from build123d import *
from build123d import SkipClean  # not in build123d's __all__

# Parameters (mm, degrees)
F0_R     = 6.1
F0_R_2   = 5
F1_DEPTH = 0.8
F2_R     = 6.1
F2_R_2   = 5.45
F3_DEPTH = 2.5
F4_R     = 5.45
F4_R_2   = 4.65
F5_DEPTH = 0.8
F7_DEPTH = 1.4
F9_DEPTH = 0.4


with BuildPart() as f1:
    # F0 (on Front) → F1 (new body)
    with BuildSketch(Plane.XZ):
        Circle(F0_R)
        Circle(F0_R_2, mode=Mode.SUBTRACT)
        Circle(F0_R_2)
    extrude(amount=F1_DEPTH)

    # F2 (on face) → F3 (join)
    with BuildSketch(Plane.XZ.offset(0.8)):
        Circle(F2_R)
        Circle(F2_R_2, mode=Mode.SUBTRACT)
    extrude(amount=F3_DEPTH)

    # F4 (on face) → F5 (join)
    with BuildSketch(Plane.XZ.offset(0.8)):
        Circle(F4_R)
        Circle(F4_R_2, mode=Mode.SUBTRACT)
    extrude(amount=F5_DEPTH)

    # F6 (on face) → F7 (cut)
    with BuildSketch(Plane.XZ.offset(3.3)):
        with BuildLine():
            Line((-1.2, -5.9808026217), (-1.6, -5.2098464469))
            ThreePointArc((-1.6, -5.2098464469), (-2.3813713563, -4.9022005735), (-3.1062049616, -4.4781682345))
            Line((-3.1062049616, -4.4781682345), (-2.555971444, -5.5386830544))
            ThreePointArc((-2.555971444, -5.5386830544), (-1.8909515594, -5.7995087895), (-1.2, -5.9808026217))
        make_face()
        with BuildLine():
            ThreePointArc((3.1062049616, -4.4781682345), (2.3813713563, -4.9022005735), (1.6, -5.2098464469))
            Line((1.6, -5.2098464469), (1.2, -5.9808026217))
            ThreePointArc((1.2, -5.9808026217), (1.8909515594, -5.7995087895), (2.555971444, -5.5386830544))
            Line((2.555971444, -5.5386830544), (3.1062049616, -4.4781682345))
        make_face()
    extrude(amount=-F7_DEPTH, mode=Mode.SUBTRACT)

    # F8 (on face) → F9 (join)
    with BuildSketch(Plane.XZ.offset(3.3)):
        with BuildLine():
            ThreePointArc((-1.6, -5.2098464469), (-2.3813713563, -4.9022005735), (-3.1062049616, -4.4781682345))
            Line((-3.1062049616, -4.4781682345), (-2.555971444, -5.5386830544))
            ThreePointArc((-2.555971444, -5.5386830544), (-1.8909515594, -5.7995087895), (-1.2, -5.9808026217))
            Line((-1.2, -5.9808026217), (-1.6, -5.2098464469))
        make_face()
        with BuildLine():
            Line((2.555971444, -5.5386830544), (3.1062049616, -4.4781682345))
            ThreePointArc((3.1062049616, -4.4781682345), (2.3813713563, -4.9022005735), (1.6, -5.2098464469))
            Line((1.6, -5.2098464469), (1.2, -5.9808026217))
            ThreePointArc((1.2, -5.9808026217), (1.8909515594, -5.7995087895), (2.555971444, -5.5386830544))
        make_face()
    with SkipClean():  # cleaning this boolean's faces spoils the solid; the shape is the same uncleaned
        extrude(amount=-F9_DEPTH)


solid = f1.part
CAD build for the part. Positions are in the model's coordinates, mm. A direction names the side the tool comes from. Give positions to 0.01 mm unless a question says otherwise; leave off trailing zeros. Write each loop counter-clockwise with the first axis right and the second up, starting at its lowest first coordinate (ties: lowest second). Pieces come first, ordered by that corner, then holes. Notation, with made-up numbers: (-25.5, 77.5) -> (17.5, 77.5) arc R38 ccw to (17.5, 115.5) -> close; hole circle Ø10 at (0, 62). An arc over 180 degrees is marked (long way). Return JSON: item names as keys, results as strings.
Item 1: Band-saw the part on D-D (x = 0). List the corners of the cut face in (y, z), then the cut area to 3 significant figures.
Answer below:
{"outline": "(-3.3, -6.1) -> (0, -6.1) -> (0, 6.1) -> (-3.3, 6.1) -> (-3.3, 5.45) -> (-1.6, 5.45) -> (-1.6, 4.65) -> (-0.8, 4.65) -> (-0.8, -4.65) -> (-1.6, -4.65) -> (-1.6, -5.45) -> (-3.3, -5.45) -> close", "area": "14.3 mm2"}
Item 2: Band-saw the part on B-B (z = 0). List the corners of the cut face in (x, y), then the cut area to 3 significant figures.
Answer below:
{"outline": "(-6.1, -3.3) -> (-5.45, -3.3) -> (-5.45, -1.6) -> (-4.65, -1.6) -> (-4.65, -0.8) -> (4.65, -0.8) -> (4.65, -1.6) -> (5.45, -1.6) -> (5.45, -3.3) -> (6.1, -3.3) -> (6.1, 0) -> (-6.1, 0) -> close", "area": "14.3 mm2"}
Item 3: Band-saw the part on C-C (x = -2.25). List the corners of the cut face in (y, z), then the cut area to 3 significant figures.
Answer below:
{"outline": "(-3.3, -5.67) -> (-2.9, -5.67) -> (-2.9, -4.96) -> (-3.3, -4.96) -> close; (-3.3, 4.96) -> (-1.6, 4.96) -> (-1.6, 4.07) -> (-0.8, 4.07) -> (-0.8, -4.07) -> (-1.6, -4.07) -> (-1.6, -4.96) -> (-1.9, -4.96) -> (-1.9, -5.67) -> (0, -5.67) -> (0, 5.67) -> (-3.3, 5.67) -> close", "area": "13.3 mm2"}
Item 4: Drill centre lines: probe 1 along Z at (x, y) = (0, -2.85); probe 2 along Z at (x, y) = (0, -1.1). Where is each one in solid material? Low to high.
Answer below:
{"probe 1": "z = -6.1 to -5.45, 5.45 to 6.1", "probe 2": "z = -6.1 to -4.65, 4.65 to 6.1"}
Item 5: Drop flat-ended pins along their axis: pin 1 (5 mm diameter, centred on x = 4.5, z = -1, fed in from +Y); pin 2 (1 mm diameter, centred on x = -3.5, z = -3, fed in from -Y); pin 3 (4.5 mm diameter, centred on x = -0.5, z = 0, fed in from -Y). Give the stop position or say it passes through.
Answer below:
{"pin 1": "stops at y = 0", "pin 2": "stops at y = -1.6", "pin 3": "stops at y = -0.8"}
Item 6: Two-plate mould, pull along X, no slides. Class faces 4 (the flat face through (-2.835, -2.407, -5.001)), 5 (the flat face through (-4, -3.3, 4)), 6 (the cylindrical face through (2.5, -1.19, 3.92)): +X half, -X half, draft (parallel to the pull), parting line (faces both ways), or undercut.
Answer below:
{"face 4": "undercut", "face 5": "draft", "face 6": "undercut"}
Item 7: Band-saw the part on A-A (y = -2.65). List the corners of the cut face in (x, z), then the cut area to 3 significant figures.
Answer below:
{"outline": "(-3.11, -4.48) arc R5.45 cw (long way) to (3.11, -4.48) -> (2.56, -5.54) arc R6.1 ccw (long way) to (-2.56, -5.54) -> close; (-1.6, -5.21) -> (-1.2, -5.98) arc R6.1 ccw to (1.2, -5.98) -> (1.6, -5.21) arc R5.45 cw to start", "area": "21.6 mm2"}
Item 8: Tool access for faces 1 (the flat face through (2.827, -2.407, -5.016)), 2 (the flat face through (0, -0.8, 0)), 3 (the flat face through (0, 0, 0)): list every direction of +Z, -Z, +X, -X, +Y, -Y with a clear straight run to the whole face (end or side of a thin tool).
Answer below:
{"face 1": "none", "face 2": "-Y", "face 3": "+Z, -Z, +X, -X, +Y"}
